Geometry check sheet. Reference: drawing and pictorial views, mm from the part's lowest x, y, z. Give positions to 0.01 mm unless a question says otherwise; leave off trailing zeros. Order: outer loops, then holes, each group sorted by start corner. A loop starts at its lowest first (then second) coordinate and runs counter-clockwise, first axis right, second up. Notation, with made-up numbers: (31, 35) -> (49, 35) arc R26 cw to (49, 63) -> close; hole circle Ø1 at (6.5, 73). An arc over 180 degrees is marked (long way). Write each question's results on one line, items separated by ' | '. Start each with the question number.
1. Cross-section at A-A, the plane y = 13.75. Enter the section's corners in (x, z) (1 decimal).
2. Cross-section at B-B, the plane z = 16.5. Enter the section's corners in (x, y) (1 decimal).
3. Mould release check, pull along Z, two halves, no side actions. Record for the marked faces 1, 2 and 3: +Z half, -Z half, draft (parallel to the pull), parting line (faces both ways), or undercut.
4. Cross-section at D-D, the plane z = 13.75. Enter the section's corners in (x, y).
5. Material ranges on L1, parallel to Z at x = 1.6, y = 17.75; L2, parallel to Y at x = 1, z = 13.5; L3, parallel to Z at x = 0.75, y = 9.5 (1 decimal), recorded low to high. Write a range as from..to.
6. Cross-section at C-C, the plane x = 1.35. State how many separate pieces and enclosed holes the cut face has, then the cut area to 3 significant figures.
7. Depth check by flat-ended pin: pin 1 Ø2 at (y, z) = (17.7, 12.75) entering from +X. Enter the tip coordinate at first touch or a pass-through.
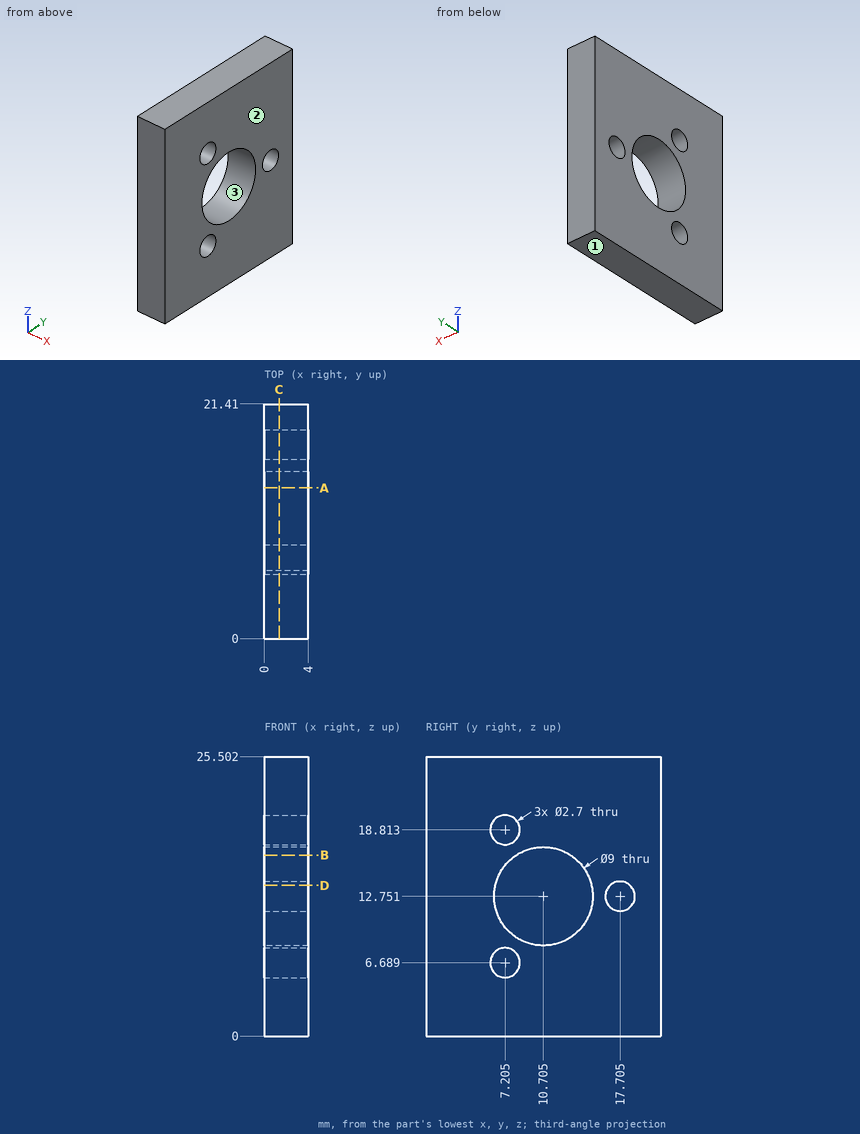
Results below:
1) outline: (0, 0) -> (4, 0) -> (4, 9.4) -> (0, 9.4) -> close; (0, 16.1) -> (4, 16.1) -> (4, 25.5) -> (0, 25.5) -> close
2) outline: (0, 0) -> (4, 0) -> (4, 8.2) -> (0, 8.2) -> close; (0, 13.2) -> (4, 13.2) -> (4, 21.4) -> (0, 21.4) -> close
3) face 1: -Z half | face 2: draft | face 3: undercut
4) outline: (0, 0) -> (4, 0) -> (4, 6.32) -> (0, 6.32) -> close; (0, 15.09) -> (4, 15.09) -> (4, 16.8) -> (0, 16.8) -> close; (0, 18.61) -> (4, 18.61) -> (4, 21.41) -> (0, 21.41) -> close
5) L1: z = 0..11.4, 14.1..25.5 | L2: y = 0..6.27, 15.14..16.58, 18.83..21.41 | L3: z = 0..8.4, 17.1..25.5
6) separate pieces: 1 | enclosed holes: 4 | area: 465 mm²
7) pin 1: passes through
